```python
from build123d import *

# Parameters (mm, degrees)
SKETCH1_W           = 130.175
SKETCH1_H           = 76.2
BOSS_EXTRUDE1_DEPTH = 20
SKETCH2_R           = 15.125
CUT_EXTRUDE1_DEPTH  = 138.102664544
SKETCH3_R           = 15.125
BOSS_EXTRUDE2_DEPTH = 4
SKETCH4_R           = 1.75
CUT_EXTRUDE2_DEPTH  = 140.31262057
CIRPATTERN1_COUNT   = 6
SKETCH5_R           = 8.5
CUT_EXTRUDE3_DEPTH  = 143.945466
SKETCH6_R           = 2.5
CUT_EXTRUDE4_DEPTH  = 88.887759564
SKETCH8_R           = 20.375
SKETCH8_R_2         = 15.375
BOSS_EXTRUDE3_DEPTH = 5
BOSS_EXTRUDE4_DEPTH = 4
BOSS_EXTRUDE5_START = -5
BOSS_EXTRUDE5_DEPTH = 10
FILLET1_R           = 10
FILLET2_R           = 3


with BuildPart() as part:
    # Sketch1 → Boss-Extrude1 (new body)
    with BuildSketch(Plane(origin=(0, 0, 0), x_dir=(1, 0, 0), z_dir=(0, 1, 0))):
        Rectangle(SKETCH1_W, SKETCH1_H)
    extrude(amount=BOSS_EXTRUDE1_DEPTH)

    # Sketch2 → Cut-Extrude1 (cut, through all)
    with BuildSketch(Plane(origin=(65.0875, 0, 0), x_dir=(0, 0, -1), z_dir=(1, 0, 0))):
        with Locations((0, 30)):
            Circle(SKETCH2_R)
    extrude(amount=-CUT_EXTRUDE1_DEPTH, mode=Mode.SUBTRACT)

    # Sketch3 → Boss-Extrude2 (add)
    with BuildSketch(Plane(origin=(65.0875, 0, 0), x_dir=(0, 0, -1), z_dir=(1, 0, 0))):
        with Locations((0, 30)):
            Circle(SKETCH3_R)
    extrude(amount=-BOSS_EXTRUDE2_DEPTH)

    # Sketch4 → Cut-Extrude2 (cut, through all)
    with BuildSketch(Plane.ZY.offset(-61.0875)):
        with Locations((0, 41)):
            Circle(SKETCH4_R)
    cut_extrude2 = extrude(amount=-CUT_EXTRUDE2_DEPTH, mode=Mode.SUBTRACT)

    # CirPattern1: Cut-Extrude2 ×6 about axis
    cirpattern1_axis = Axis((0, 30, 0), (1, 0, 0))
    for i in range(1, CIRPATTERN1_COUNT):
        add(cut_extrude2.rotate(cirpattern1_axis, i * 360 / CIRPATTERN1_COUNT), mode=Mode.SUBTRACT)

    # Sketch5 → Cut-Extrude3 (cut, through all)
    with BuildSketch(Plane(origin=(65.0875, 0, 0), x_dir=(0, 0, -1), z_dir=(1, 0, 0))):
        with Locations((0, 30)):
            Circle(SKETCH5_R)
    extrude(amount=-CUT_EXTRUDE3_DEPTH, mode=Mode.SUBTRACT)

    # Sketch6 → Cut-Extrude4 (cut, through all)
    with BuildSketch(Plane.XZ):
        with Locations(Location((60.7695, 23.368, 0), (0, 0, 270))):
            Circle(SKETCH6_R)
        with Locations(Location((60.7695, -27.432, 0), (0, 0, 270))):
            Circle(SKETCH6_R)
    cut_extrude4 = extrude(amount=-CUT_EXTRUDE4_DEPTH, mode=Mode.SUBTRACT)

    # Mirror1: Cut-Extrude4 across plane
    add(cut_extrude4.mirror(Plane(origin=(0, 0, 0), x_dir=(0, 0, 1), z_dir=(1, 0, 0))), mode=Mode.SUBTRACT)

    # Sketch8 → Boss-Extrude3 (add, symmetric)
    with BuildSketch(Plane(origin=(10, 0, 0), x_dir=(0, 0, -1), z_dir=(1, 0, 0))):
        with Locations((0, 30)):
            Circle(SKETCH8_R)
        with Locations((0, 30)):
            Circle(SKETCH8_R_2, mode=Mode.SUBTRACT)
    extrude(amount=BOSS_EXTRUDE3_DEPTH, both=True)

    # Sketch9 → Boss-Extrude4 (add)
    with BuildSketch(Plane(origin=(65.0875, 0, 0), x_dir=(0, 0, -1), z_dir=(1, 0, 0))):
        with BuildLine():
            ThreePointArc((-11.347494217, 20), (-14.149142642, 24.655153184), (-15.125, 30))
            Line((-15.125, 30), (-15.125, 20))
            Line((-15.125, 20), (-11.347494217, 20))
        make_face()
        with BuildLine():
            Line((15.125, 20), (15.125, 30))
            ThreePointArc((15.125, 30), (14.149142642, 24.655153184), (11.347494217, 20))
            Line((11.347494217, 20), (15.125, 20))
        make_face()
    extrude(amount=-BOSS_EXTRUDE4_DEPTH)

    # Sketch10 → Boss-Extrude5 (add)
    with BuildSketch(Plane(origin=(10, 0, 0), x_dir=(0, 0, -1), z_dir=(1, 0, 0)).offset(BOSS_EXTRUDE5_START)):
        with BuildLine():
            ThreePointArc((-17.752200568, 20), (-19.708395566, 24.83088313), (-20.375, 30))
            Line((-20.375, 30), (-20.375, 20))
            Line((-20.375, 20), (-17.752200568, 20))
        make_face()
        with BuildLine():
            Line((20.375, 20), (20.375, 30))
            ThreePointArc((20.375, 30), (19.708395566, 24.83088313), (17.752200568, 20))
            Line((17.752200568, 20), (20.375, 20))
        make_face()
    extrude(amount=BOSS_EXTRUDE5_DEPTH)

    # Fillet1
    fillet1_edges = [part.edges().sort_by_distance(p)[0] for p in [
        (10, 20, -20.375),
        (10, 20, 20.375),
    ]]
    fillet(fillet1_edges, radius=FILLET1_R - 0.0001)  # a hair under: the kernel refuses the full size

    # Fillet2
    fillet2_edges = [part.edges().sort_by_distance(p)[0] for p in [
        (63.0875, 20, 15.125),
        (63.0875, 20, -15.125),
    ]]
    fillet(fillet2_edges, radius=FILLET2_R)


solid = part.part
```
Check sheet for the modelled part. Datum: model origin and axes. Units: mm. A direction names the side the tool comes from. Give positions to 0.01 mm unless a question says otherwise; leave off trailing zeros. Loops run counter-clockwise (first coordinate to the right, second up) from the corner with the lowest first, then second, coordinate; pieces in that order, holes last. Notation, with made-up numbers: M 4,1 L 28,1 A30 ccw 28,23 Z; hole C -34,-11 d8. An arc over 180 degrees is marked long. Answer in a Markdown table with one row per item.
1) Depth check by flat-ended pin: pin 1 (3 mm diameter, centred on y = 25, z = 16.5, fed in from +X); pin 2 (15 mm diameter, centred on y = 34.5, z = 7.5, fed in from -X); pin 3 (8 mm diameter, centred on x = -60.77, z = -27.43, fed in from +Y); pin 4 (18.5 mm diameter, centred on y = 30, z = 0, fed in from -X). Enter the tip coordinate at first touch or a pass-through.
Solutions:
| item | result |
|---|---|
| pin 1 | stops at x = 65.09 |
| pin 2 | stops at x = 5 |
| pin 3 | stops at y = 20 |
| pin 4 | stops at x = 61.09 |
2) Cross-section at B-B (y = 24.5). Enter the section's corners in (x, z) (1 decimal), plus the area to 3 significant figures.
Solutions:
| item | result |
|---|---|
| outline | M 5,-22 L 15,-22 L 15,-14.4 L 5,-14.4 Z; M 5,14.4 L 15,14.4 L 15,22 L 5,22 Z; M 61.1,-15.1 L 65.1,-15.1 L 65.1,-11.3 L 61.1,-11.3 Z; M 61.1,-7.8 L 65.1,-7.8 L 65.1,-6.5 L 61.1,-6.5 Z; M 61.1,6.5 L 65.1,6.5 L 65.1,7.8 L 61.1,7.8 Z; M 61.1,11.3 L 65.1,11.3 L 65.1,15.1 L 61.1,15.1 Z |
| area | 194 mm^2 |
3) Thickness scan on line 1 (Z direction, x = 9, y = 30) (3 decimals); line 2 (Z direction, x = 63, y = 24) (3 decimals); line 3 (Y direction, x = 14, z = 32.5). Record the ranges inside material, lowest first.
Solutions:
| item | result |
|---|---|
| line 1 | z = -20.375 to -15.375, 15.375 to 20.375 |
| line 2 | z = -15.125 to -11.203, -7.849 to -6.021, 6.021 to 7.849, 11.203 to 15.125 |
| line 3 | y = 0 to 20 |
4) Cross-section at D-D (y = 41). Enter the section's corners in (x, z).
Solutions:
| item | result |
|---|---|
| outline | M 5,-17.15 L 15,-17.15 L 15,-10.74 L 5,-10.74 Z; M 5,10.74 L 15,10.74 L 15,17.15 L 5,17.15 Z; M 61.09,-10.38 L 65.09,-10.38 L 65.09,-1.75 L 61.09,-1.75 Z; M 61.09,1.75 L 65.09,1.75 L 65.09,10.38 L 61.09,10.38 Z |
5) Mould release check, pull along X, two halves, no side actions. Record for faces 1 (the face through (63.25, 9.86, -27.11)), 2 (the face through (-63.25, 9.86, -27.11)), 3 (the face through (-65.088, 10, 1)), 4 (the face through (-1.117, 14.876, 0.18)): released by +X, released by -X, zero draft, split by the parting line, or undercut.
Solutions:
| item | result |
|---|---|
| face 1 | undercut |
| face 2 | undercut |
| face 3 | released by -X |
| face 4 | zero draft |
6) Tool access check on faces 5 (the face through (63, 27, 15.125)), 6 (the face through (10.07, 23.007, 23.227)), 7 (the face through (63.06, 20.855, -16.027)). Record the directions out of +Z, -Z, +X, -X, +Y, -Y that give a thin tool (end or side, any length) a straight path to the whole face; none if there is none.
Solutions:
| item | result |
|---|---|
| face 5 | +Z, +X, +Y |
| face 6 | +Z, +X, -X, +Y |
| face 7 | -Z, +X, +Y |
7) Cross-section at A-A (z = 0). Count the separate pieces of the cut face and the enclosed holes in it, plus the area to 3 significant figures.
Solutions:
| item | result |
|---|---|
| separate pieces | 5 |
| enclosed holes | 0 |
| area | 2,010 mm^2 |
